Input: part model. Units: mm. Frame: model coordinates. A direction names the side the tool comes from. Coordinates: 2 decimals unless noted, no trailing zeros. Loops run counter-clockwise (first coordinate to the right, second up) from the corner with the lowest first, then second, coordinate; pieces in that order, holes last. Notation, with made-up numbers: M 72,-12 L 82,-12 A5 cw 82,-7 Z; hole C 39.25,-23.75 d7. An arc over 180 degrees is marked long. Use a Markdown table: item, result. Add a question column.
1. Draft query along X for faces 4 (the flat face through (52.7, 34, 33)), 5 (the flat face through (31, 30, 30)), 6 (the flat face through (37.7, 18, 15)), 7 (the flat face through (45, 42, 0)). Return one class per face: +X half, -X half, draft (parallel to the pull), parting line (faces both ways), or undercut.
2. Section A-A on x = 32. Output: boundary loops of the cut face in (y, z), then the cut area to 3 significant figures.
3. Set-up query: faces 1 (the flat face through (31, 45, 60)), 2 (the flat face through (45, 35, 15)), 3 (the flat face through (13.333, 47, 77)). Return all of +Z, -Z, +X, -X, +Y, -Y with unobstructed straight access to the full face (end or side cutting, diameter ignored); none if empty.
4. Section C-C on y = 26. Output: boundary loops of the cut face in (x, z), then the cut area to 3 significant figures.
5. Pin query (flat end, axial travel): pin 1 (4 mm diameter, centred on x = 24.5, y = 39, fed in from +Z); pin 2 (3 mm diameter, centred on x = 35.5, y = 47, fed in from -Z); pin 3 (3 mm diameter, centred on y = 27, z = 10.5, fed in from +X); pin 4 (20.5 mm diameter, centred on x = 26.5, z = 51, fed in from -Y). Return the tip coordinate at first contact, or that it passes through.
6. Line query: L1, parallel to Y at x = 24, z = 22; L2, parallel to X at y = 46, z = 5; L3, parallel to Y at x = 20.5, z = 69. Output: solid intervals per line, ascending. Write a range as [from, to].
7. Section B-B on z = 79. Output: boundary loops of the cut face in (x, y).
8. Section D-D on z = 17.5. Output: boundary loops of the cut face in (x, y), then the cut area to 3 significant figures.
```python
from build123d import *

# Parameters (mm, degrees)
F0_W     = 15
F0_H     = 15
F1_DEPTH = 30
F2_W     = 42.7
F2_H     = 40
F3_DEPTH = 5
F4_W     = 42.7
F4_H     = 5
F5_DEPTH = 50
F6_W     = 35.6923062354
F6_H     = 6.7692324519
F7_DEPTH = 25
F8_R     = 1


with BuildPart() as f1:
    # F0 (on Top) → F1 (new body)
    with BuildSketch(Plane.XY):
        with Locations((17.5, 17.5)):
            Rectangle(F0_W, F0_H)
    extrude(amount=F1_DEPTH)



with BuildPart() as f1b:
    # F0 (on Top) → F1, piece 2 (new body)
    with BuildSketch(Plane.XY):
        with Locations((17.5, 42.5)):
            Rectangle(F0_W, F0_H)
    extrude(amount=F1_DEPTH)


with BuildPart() as f1c:
    # F0 (on Top) → F1, piece 3 (new body)
    with BuildSketch(Plane.XY):
        with Locations((45.2, 17.5)):
            Rectangle(F0_W, F0_H)
    extrude(amount=F1_DEPTH)


with BuildPart() as f1d:
    # F0 (on Top) → F1, piece 4 (new body)
    with BuildSketch(Plane.XY):
        with Locations((45.2, 42.5)):
            Rectangle(F0_W, F0_H)
    extrude(amount=F1_DEPTH)


with BuildPart() as f1_1:
    add(f1.part)

    add(f1b.part)  # F3 merges F1b

    add(f1c.part)  # F3 merges F1c

    add(f1d.part)  # F3 merges F1d
    # F2 (on face) → F3 (join)
    with BuildSketch(Plane.XY.offset(30)):
        with Locations((31.35, 30)):
            Rectangle(F2_W, F2_H)
    extrude(amount=F3_DEPTH)

    # F4 (on face) → F5 (join)
    with BuildSketch(Plane.XY.offset(35)):
        with Locations((31.35, 47.5)):
            Rectangle(F4_W, F4_H)
    extrude(amount=F5_DEPTH)

    # F6 (on face) → F7 (cut)
    with BuildSketch(Plane(origin=(0, 50, 0), x_dir=(-1, 0, 0), z_dir=(0, 1, 0))):
        with Locations((-31.1794867739, 76.5897445381)):
            Rectangle(F6_W, F6_H)
    extrude(amount=-F7_DEPTH, mode=Mode.SUBTRACT)

    # F8
    f8_edges = [f1_1.edges().sort_by_distance(p)[0] for p in [
        (52.7, 27.5, 35),
        (31.35, 10, 35),
        (10, 27.5, 35),
        (31.35, 45, 35),
        (31.35, 50, 85),
        (10, 47.5, 85),
        (31.35, 45, 85),
        (52.7, 47.5, 85),
        (37.7, 10, 15),
        (31.35, 10, 30),
        (25, 10, 15),
        (17.5, 10, 0),
        (10, 10, 17.5),
        (52.7, 10, 17.5),
        (45.2, 10, 0),
        (52.7, 35, 15),
        (52.7, 30, 30),
        (52.7, 25, 15),
        (52.7, 17.5, 0),
        (52.7, 45, 60),
        (52.7, 50, 42.5),
        (52.7, 42.5, 0),
        (45.2, 50, 0),
        (10, 50, 42.5),
        (37.7, 50, 15),
        (17.5, 50, 0),
        (31.35, 50, 30),
        (25, 50, 15),
        (13.333334, 50, 76.589745),
        (31.179487, 50, 73.205128),
        (49.02564, 50, 76.589745),
        (31.179487, 50, 79.974361),
        (10, 45, 60),
    ]]
    fillet(f8_edges, radius=F8_R)


solid = f1_1.part
```
Answers below:
| question | item | result |
|---|---|---|
| 1 | face 4 | +X half |
| 1 | face 5 | undercut |
| 1 | face 6 | undercut |
| 1 | face 7 | draft |
| 2 | outline | M 10,31 A1 ccw 11,30 L 49,30 A1 ccw 50,31 L 50,72.21 A1 ccw 49,73.21 L 45,73.21 L 45,36 A1 cw 44,35 L 11,35 A1 ccw 10,34 Z; M 45,79.97 L 49,79.97 A1 ccw 50,80.97 L 50,84 A1 ccw 49,85 L 46,85 A1 ccw 45,84 Z |
| 2 | area | 415 mm² |
| 3 | face 1 | +Z, +X, -X, -Y |
| 3 | face 2 | -Z, +X, -X |
| 3 | face 3 | +Y, -Y |
| 4 | outline | M 10,30 L 51.7,30 A1 ccw 52.7,31 L 52.7,34 A1 ccw 51.7,35 L 11,35 A1 ccw 10,34 Z |
| 4 | area | 213 mm² |
| 5 | pin 1 | stops at z = 35 |
| 5 | pin 2 | stops at z = 30 |
| 5 | pin 3 | passes through |
| 5 | pin 4 | stops at y = 45 |
| 6 | L1 | y = [10, 25], [35, 50] |
| 6 | L2 | x = [10, 25], [37.7, 52.7] |
| 6 | L3 | y = [45, 50] |
| 7 | outline | M 10,46 A1 ccw 11,45 L 13.33,45 L 13.33,49 A1 ccw 12.33,50 L 11,50 A1 ccw 10,49 Z; M 49.03,45 L 51.7,45 A1 ccw 52.7,46 L 52.7,49 A1 ccw 51.7,50 L 50.03,50 A1 ccw 49.03,49 Z |
| 8 | outline | M 10,11 A1 ccw 11,10 L 24,10 A1 ccw 25,11 L 25,25 L 10,25 Z; M 10,35 L 25,35 L 25,49 A1 ccw 24,50 L 11,50 A1 ccw 10,49 Z; M 37.7,11 A1 ccw 38.7,10 L 51.7,10 A1 ccw 52.7,11 L 52.7,24 A1 ccw 51.7,25 L 37.7,25 Z; M 37.7,35 L 51.7,35 A1 ccw 52.7,36 L 52.7,49 A1 ccw 51.7,50 L 38.7,50 A1 ccw 37.7,49 Z |
| 8 | area | 898 mm² |
